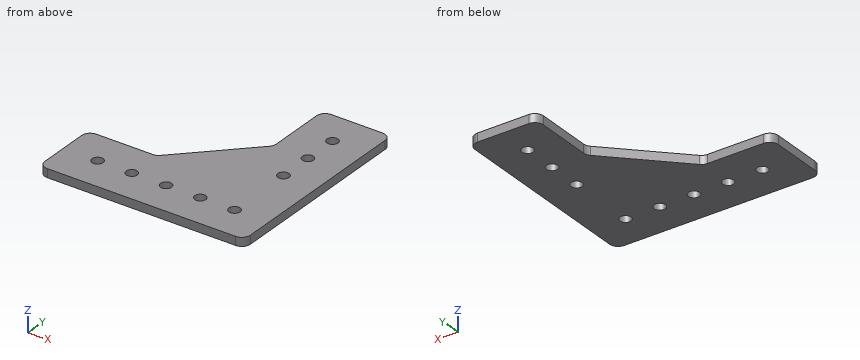
Autodesk Inventor part; units mm, degrees
ref_plane "YZ Plane" through (0, 0, 0) normal (1, 0, 0) x (0, 1, 0)
ref_plane "XZ Plane" through (0, 0, 0) normal (0, 1, 0) x (-1, 0, 0)
ref_plane "XY Plane" through (0, 0, 0) normal (0, 0, 1) x (1, 0, 0)
sketch "Sketch1" plane through (0, 0, 0) normal (0, 0, 1) x (1, 0, 0)
  line L0 (-32.8613, -32.8613) -> (43.3387, -32.8613)
  line L1 (43.3387, -32.8613) -> (43.3387, 43.3387)
  line L2 (-32.8613, -32.8613) -> (43.3387, 43.3387) construction
  line L3 (43.3387, 43.3387) -> (-32.8613, -32.8613)
  line L4 (43.3387, 43.3387) -> (17.9387, 43.3387)
  line L5 (17.9387, 43.3387) -> (17.9387, 17.9387)
  line L6 (43.3387, 22.2601) -> (43.3387, 43.3387)
  line L7 (-32.8613, -32.8613) -> (-7.4613, -32.8613)
  line L8 (-7.4613, -32.8613) -> (-7.4613, -7.4613)
  line L9 (-7.4613, -7.4613) -> (-32.8613, -7.4613)
  line L10 (-32.8613, -7.4613) -> (-32.8613, -32.8613)
  point P0 (0, 0)
  dimension "d1" = 76.2
  dimension "d2" = 76.2
  dimension "d7" = 25.4
  dimension "d8" = 25.4
extrude "Extrusion1" add sketch "Sketch1" along normal blind 3.175
fillet "Fillet2" radius 3.175 7 edges at (17.9387, 43.3387, 1.5875) (43.3387, 43.3387, 1.5875) (17.9387, 17.9387, 1.5875) (-7.4613, -7.4613, 1.5875) (-32.8613, -7.4613, 1.5875) (-32.8613, -32.8613, 1.5875) (43.3387, -32.8613, 1.5875)
sketch "Sketch2" plane through (0, 0, 3.175) normal (0, 0, 1) x (1, 0, 0)
  arc A0 (20.0074, -20.0851) -> (15.8701, -20.0851) centre (17.9387, -20.1613) ccw
  line L0 (20.0074, -20.0851) -> (28.5701, -20.0851)
  arc A1 (32.7074, -20.0851) -> (28.5701, -20.0851) centre (30.6387, -20.1613) ccw
  line L1 (32.7074, -20.0851) -> (43.3387, -20.0851)
  line L2 (43.3387, -20.0851) -> (43.3387, -7.4613)
  line L3 (-693.2613, -7.4613) -> (43.3387, -7.4613)
  line L4 (-693.2613, -7.4613) -> (-693.2613, -20.0851)
  line L5 (-693.2613, -20.0851) -> (-682.6299, -20.0851)
  arc A2 (-678.4926, -20.0851) -> (-682.6299, -20.0851) centre (-680.5613, -20.1613) ccw
  line L6 (-678.4926, -20.0851) -> (-669.9299, -20.0851)
  arc A3 (-665.7926, -20.0851) -> (-669.9299, -20.0851) centre (-667.8613, -20.1613) ccw
  line L7 (-665.7926, -20.0851) -> (-657.2299, -20.0851)
  arc A4 (-653.0926, -20.0851) -> (-657.2299, -20.0851) centre (-655.1613, -20.1613) ccw
  line L8 (-653.0926, -20.0851) -> (-644.5299, -20.0851)
  arc A5 (-640.3926, -20.0851) -> (-644.5299, -20.0851) centre (-642.4613, -20.1613) ccw
  line L9 (-640.3926, -20.0851) -> (-631.8299, -20.0851)
  arc A6 (-627.6926, -20.0851) -> (-631.8299, -20.0851) centre (-629.7613, -20.1613) ccw
  line L10 (-627.6926, -20.0851) -> (-272.9448, -20.0851)
  arc A7 (-242.32, -20.0851) -> (-272.9448, -20.0851) centre (-257.6324, -29.1216) ccw
  line L11 (-242.32, -20.0851) -> (-22.2299, -20.0851)
  arc A8 (-18.0926, -20.0851) -> (-22.2299, -20.0851) centre (-20.1613, -20.1613) ccw
  line L12 (-18.0926, -20.0851) -> (-9.5299, -20.0851)
  arc A9 (-5.3926, -20.0851) -> (-9.5299, -20.0851) centre (-7.4613, -20.1613) ccw
  line L13 (-5.3926, -20.0851) -> (3.1701, -20.0851)
  arc A10 (7.3074, -20.0851) -> (3.1701, -20.0851) centre (5.2387, -20.1613) ccw
  line L14 (7.3074, -20.0851) -> (15.8701, -20.0851)
  arc A11 (-84.7976, -15.8974) -> (-84.7976, -10.792) centre (-84.7976, -13.3447) ccw
  line L15 (-84.7976, -15.8974) -> (-94.3226, -15.8974)
  arc A12 (-94.3226, -10.792) -> (-94.3226, -15.8974) centre (-94.3226, -13.3447) ccw
  line L16 (-94.3226, -10.792) -> (-84.7976, -10.792)
  arc A13 (-604.3151, -10.792) -> (-604.3151, -15.8974) centre (-604.3151, -13.3447) ccw
  line L17 (-604.3151, -10.792) -> (-594.7901, -10.792)
  arc A14 (-594.7901, -15.8974) -> (-594.7901, -10.792) centre (-594.7901, -13.3447) ccw
  line L18 (-594.7901, -15.8974) -> (-604.3151, -15.8974)
  arc A15 (-564.9959, -10.792) -> (-564.9959, -15.8974) centre (-564.9959, -13.3447) ccw
  line L19 (-564.9959, -10.792) -> (-555.4709, -10.792)
  arc A16 (-555.4709, -15.8974) -> (-555.4709, -10.792) centre (-555.4709, -13.3447) ccw
  line L20 (-555.4709, -15.8974) -> (-564.9959, -15.8974)
  arc A17 (-55.0034, -10.792) -> (-55.0034, -15.8974) centre (-55.0034, -13.3447) ccw
  line L21 (-55.0034, -10.792) -> (-45.4784, -10.792)
  arc A18 (-45.4784, -15.8974) -> (-45.4784, -10.792) centre (-45.4784, -13.3447) ccw
  line L22 (-45.4784, -15.8974) -> (-55.0034, -15.8974)
  arc A19 (30.7149, 28.5701) -> (30.7149, 32.7074) centre (30.6387, 30.6387) ccw
  line L23 (30.7149, 20.0074) -> (30.7149, 28.5701)
  arc A20 (30.7149, 15.8701) -> (30.7149, 20.0074) centre (30.6387, 17.9387) ccw
  line L24 (30.7149, 7.3074) -> (30.7149, 15.8701)
  arc A21 (30.7149, 3.1701) -> (30.7149, 7.3074) centre (30.6387, 5.2387) ccw
  line L25 (30.7149, -7.4613) -> (30.7149, 3.1701)
  line L26 (43.3387, -7.4613) -> (30.7149, -7.4613)
  line L27 (43.3387, 221.1387) -> (43.3387, -7.4613)
  line L28 (43.3387, 221.1387) -> (30.7149, 221.1387)
  line L29 (30.7149, 190.6448) -> (30.7149, 221.1387)
  arc A22 (30.7149, 183.509) -> (30.7149, 190.6448) centre (30.6387, 187.0769) ccw
  line L30 (30.7149, 32.7074) -> (30.7149, 183.509)
  point P0 (0, 0)
  point P1 (30.6387, 5.2387)
  point P2 (30.6387, 30.6387)
hole "Hole1" at (30.6387, 30.6387, 3.175) at (30.6387, 5.2387, 3.175) at (30.6387, -20.1613, 3.175) at (5.2387, -20.1613, 3.175) at (-20.1613, -20.1613, 3.175) at (-7.4613, -20.1613, 3.175) at (17.9387, -20.1613, 3.175) at (30.6387, 17.9387, 3.175) direction (0, 0, -1) diameter 4.1402 end through all
properties part number "C21_TK_TriangleGusset" material "Aluminum 6061"
For this review, take the finished solid that the model builds, in its own axes (mm). Give positions to 0.01 mm unless a question says otherwise; leave off trailing zeros. Write each loop counter-clockwise with the first axis right and the second up, starting at its lowest first coordinate (ties: lowest second). Pieces come first, ordered by that corner, then holes. Notation, with made-up numbers: M -26,74 L -18,74 A17 ccw -18,82 Z; hole C 39,21.5 d2. An arc over 180 degrees is marked long. One line per item, written item: value.
1) For P1, Ø5, axis at x = 30.64, y = 5.24, coming from the -Z side; P2, Ø3.5, axis at x = 17.94, y = -20.16, coming from the +Z side; P3, Ø1.6, axis at x = -17.5, z = 2, coming from the +Y side; P4, Ø1, axis at y = 12.5, z = 1, coming from the -X side, all flat-tipped, find the tip position at first contact; note any pin that passes through.
Results are:
P1: stops at z = 0
P2: passes through
P3: stops at y = -7.46
P4: stops at x = 12
2) Take a section at C-C, the plane y = 24.5. Write out the cut boundary in (x, z) (3 decimals), then the cut area to 3 significant figures.
Results are:
outline: M 17.939,0 L 43.339,0 L 43.339,3.175 L 17.939,3.175 Z
area: 80.6 mm²
3) For line 1 (X direction, y = -20, z = 2.75); line 2 (Y direction, x = 31.5, z = 2.25); line 3 (X direction, y = 27, z = 1.6), list the stretches that pass through material, from the lowest coordinate up. Write a range as from..to.
Results are:
line 1: x = -32.86..-22.23, -18.1..-9.53, -5.4..3.17, 7.3..15.87, 20..28.57, 32.7..43.34
line 2: y = -32.86..-22.04, -18.28..3.36, 7.12..16.06, 19.82..28.76, 32.52..43.34
line 3: x = 17.94..43.34
4) Take a section at B-B, the plane y = -20. Write out the cut boundary in (x, z) (1 decimal).
Results are:
outline: M -32.9,0 L -22.2,0 L -22.2,3.2 L -32.9,3.2 Z; M -18.1,0 L -9.5,0 L -9.5,3.2 L -18.1,3.2 Z; M -5.4,0 L 3.2,0 L 3.2,3.2 L -5.4,3.2 Z; M 7.3,0 L 15.9,0 L 15.9,3.2 L 7.3,3.2 Z; M 20,0 L 28.6,0 L 28.6,3.2 L 20,3.2 Z; M 32.7,0 L 43.3,0 L 43.3,3.2 L 32.7,3.2 Z
5) Take a section at A-A, the plane z = 2.35. Count the separate pieces of the cut face and the enclosed holes in it, then the cut area to 3 significant figures.
Results are:
separate pieces: 1
enclosed holes: 8
area: 3,430 mm²
6) Take a section at D-D, the plane y = -0.5. Write out the cut boundary in (x, z) (3 decimals), then the cut area to 3 significant figures.
Results are:
outline: M -0.5,0 L 43.339,0 L 43.339,3.175 L -0.5,3.175 Z
area: 139 mm²
